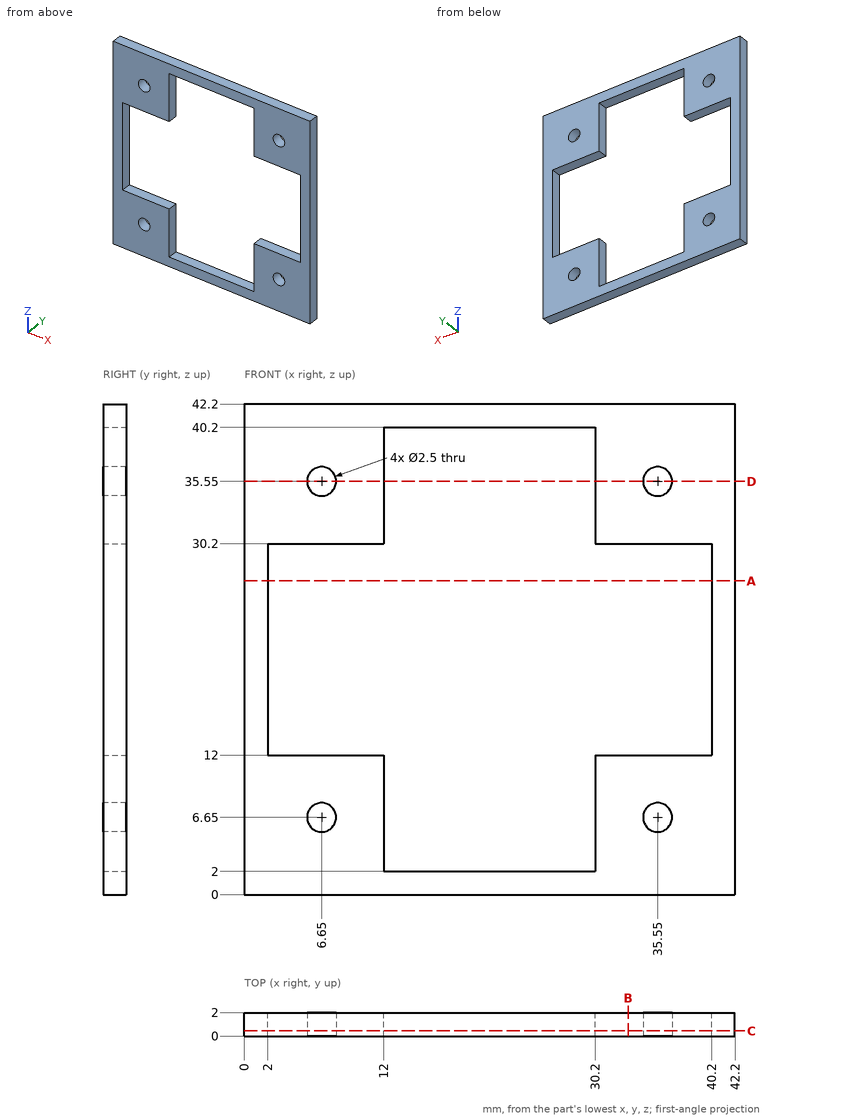
Geometry: see drawing. Coordinates: mm, zero at the bounding-box minimum. Coordinates: 2 decimals unless noted, no trailing zeros. Order: outer loops, then holes, each group sorted by start corner. A loop starts at its lowest first (then second) coordinate and runs counter-clockwise, first axis right, second up. Notation, with made-up numbers: (-33, 10) - (-5, 10) arc R24 ccw to (-5, 21) - close; hole circle Ø4 at (63, 84). An arc over 180 degrees is marked (long way). Write each question's results on one line, items separated by ' | '.
1) Line query: line 1 (X direction, y = 1.5, z = 35.55); line 2 (Z direction, x = 21.5, y = 1.7). Output: solid intervals per line, ascending. Write a range as from..to.
Results list:
line 1: 0..5.4, 7.9..12, 30.2..34.3, 36.8..42.2 | line 2: 0..2, 40.2..42.2
2) Section A-A, the plane z = 27. Return loops of the section in (x, y).
Results list:
outline: (0, 0) - (2, 0) - (2, 2) - (0, 2) - close; (40.2, 0) - (42.2, 0) - (42.2, 2) - (40.2, 2) - close
3) Section C-C, the plane y = 0.45. Return loops of the section in (x, z).
Results list:
outline: (0, 0) - (42.2, 0) - (42.2, 42.2) - (0, 42.2) - close; hole (2, 12) - (12, 12) - (12, 2) - (30.2, 2) - (30.2, 12) - (40.2, 12) - (40.2, 30.2) - (30.2, 30.2) - (30.2, 40.2) - (12, 40.2) - (12, 30.2) - (2, 30.2) - close; hole circle Ø2.5 at (6.65, 6.65); hole circle Ø2.5 at (6.65, 35.55); hole circle Ø2.5 at (35.55, 6.65); hole circle Ø2.5 at (35.55, 35.55)
4) Section B-B, the plane x = 33. Return loops of the section in (y, z), plus the area to 3 significant figures.
Results list:
outline: (0, 0) - (2, 0) - (2, 12) - (0, 12) - close; (0, 30.2) - (2, 30.2) - (2, 42.2) - (0, 42.2) - close | area: 48.0 mm^2
5) Section D-D, the plane z = 35.55. Return loops of the section in (x, y).
Results list:
outline: (0, 0) - (5.4, 0) - (5.4, 2) - (0, 2) - close; (7.9, 0) - (12, 0) - (12, 2) - (7.9, 2) - close; (30.2, 0) - (34.3, 0) - (34.3, 2) - (30.2, 2) - close; (36.8, 0) - (42.2, 0) - (42.2, 2) - (36.8, 2) - close
